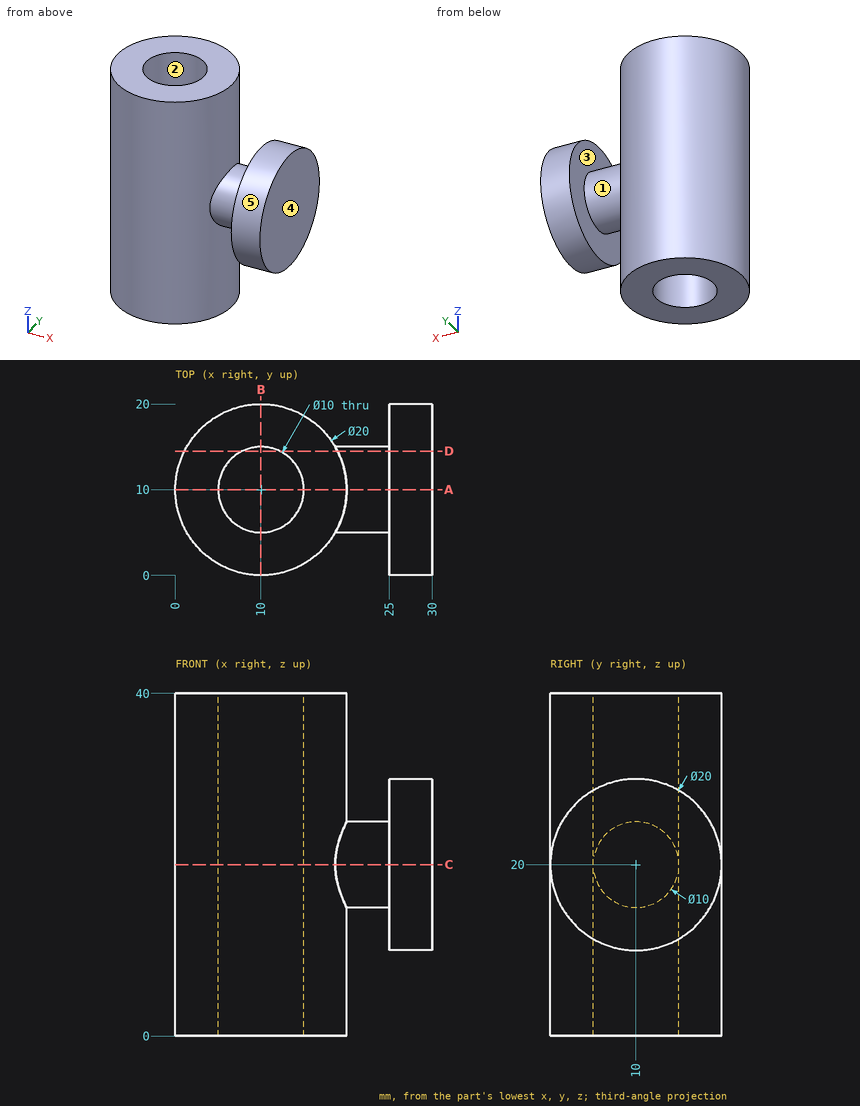
Answer from the drawing. Dimensions are ordinates in mm from the lowest x, y and z of the part. A direction names the side the tool comes from. Round coordinates to 2 decimals unless told otherwise and drop trailing zeros. Order: outer loops, then holes, each group sorted by start corner. A loop starts at its lowest first (then second) coordinate and runs counter-clockwise, first axis right, second up.
1) The part is cut by section D-D on y = 14.5. Write down the section's boundary in (x, z).
2) The part is cut by section C-C on z = 20. Write down the section's boundary in (x, y).
3) Flat-ended cylindrical pins translate along their axes: pin 1 (10 mm diameter, centred on x = 4.5, z = 19.5, fed in from +Y); pin 2 (1 mm diameter, centred on x = 25.5, z = 13, fed in from -Y); pin 3 (1 mm diameter, centred on y = 13.5, z = 21, fed in from -X). Find the tip coordinate at first contact, or state that the pin passes through.
4) The part is cut by section A-A on y = 10. Write down the section's boundary in (x, z), plus the area to 3 significant figures.
5) For the marked faces 4 and 5, determine the directions among +Z, -Z, +X, -X, +Y, -Y from which every point of the face is accessible in a straight line to the end or side of a thin tool.
6) Straight lines are drawn through the part: L1, parallel to Y at x = 10, z = 30; L2, parallel to X at y = 12.25, z = 14; L3, parallel to X at y = 6.25, z = 28.5. For each, find the intervals that lie inside material, in ascending order.
7) The mould has two halves that part along Y. Classify the marked faces 1, 2 and 3: released by +Y, released by -Y, zero draft, split by the parting line, or undercut.
8) The part is cut by section B-B on x = 10. Write down the section's boundary in (y, z).
Resolved:
1. outline: (1.07, 0) - (7.82, 0) - (7.82, 40) - (1.07, 40) - close; (12.18, 0) - (18.93, 0) - (18.93, 17.82) - (25, 17.82) - (25, 11.07) - (30, 11.07) - (30, 28.93) - (25, 28.93) - (25, 22.18) - (18.93, 22.18) - (18.93, 40) - (12.18, 40) - close
2. outline: (18.66, 5) - (25, 5) - (25, 0) - (30, 0) - (30, 20) - (25, 20) - (25, 15) - (18.66, 15) arc R10 ccw (long way) to start; hole circle Ø10 at (10, 10)
3. pin 1: stops at y = 19.99
3. pin 2: stops at y = 2.4
3. pin 3: stops at x = 0.46
4. outline: (0, 0) - (5, 0) - (5, 40) - (0, 40) - close; (15, 0) - (20, 0) - (20, 15) - (25, 15) - (25, 10) - (30, 10) - (30, 30) - (25, 30) - (25, 25) - (20, 25) - (20, 40) - (15, 40) - close
4. area: 550 mm2
5. face 4: +Z, -Z, +X, +Y, -Y
5. face 5: +X
6. L1: y = 0 to 5, 15 to 20
6. L2: x = 0.26 to 5.53, 14.47 to 19.74, 25 to 30
6. L3: x = 0.73 to 6.69, 13.31 to 19.27, 25 to 30
7. face 1: split by the parting line
7. face 2: undercut
7. face 3: zero draft
8. outline: (0, 0) - (5, 0) - (5, 40) - (0, 40) - close; (15, 0) - (20, 0) - (20, 40) - (15, 40) - close
